Geometry: final body of the model. Coordinates: model frame, mm. A direction names the side the tool comes from. Round coordinates to 2 decimals unless told otherwise and drop trailing zeros. Answer in a Markdown table with one row per item.
Autodesk Inventor part; units mm, degrees
ref_plane "C1_XY" through (0, 0, 0) normal (0, 0, 1) x (1, 0, 0)
ref_plane "C1_YZ" through (0, 0, 0) normal (1, 0, 0) x (0, 1, 0)
ref_plane "C1_ZX" through (0, 0, 0) normal (0, 1, 0) x (0, 0, 1)
sketch "Sketch_63" plane through (0, 0, 0) normal (0, 0, 1) x (1, 0, 0)
  line L0 (-10, -7) -> (-8, -7)
  line L1 (-8, -7) -> (-8, -4)
  line L2 (-8, -4) -> (-7.0607, -4)
  line L3 (-7.0607, -4) -> (-4, -7.0607)
  line L4 (-4, -7.0607) -> (-4, -9.4804)
  line L5 (-4, -9.4804) -> (-3.7, -10)
  line L6 (-3.7, -10) -> (-4, -10.5196)
  line L7 (-4, -10.5196) -> (-4, -12.9393)
  line L8 (-4, -12.9393) -> (-7.0607, -16)
  line L9 (-7.0607, -16) -> (-8, -16)
  line L10 (-8, -16) -> (-8, -13)
  line L11 (-8, -13) -> (-10, -13)
  line L12 (-10, -13) -> (-10, -19)
  arc A0 (-10, -19) -> (-9, -20) centre (-9, -19) ccw
  line L13 (-9, -20) -> (-3, -20)
  line L14 (-3, -20) -> (-3, -18)
  line L15 (-3, -18) -> (-6, -18)
  line L16 (-6, -18) -> (-6, -17.0607)
  line L17 (-6, -17.0607) -> (-2.9393, -14)
  line L18 (-2.9393, -14) -> (-0.5196, -14)
  line L19 (-0.5196, -14) -> (0, -13.7)
  line L20 (0, -13.7) -> (0.5196, -14)
  line L21 (0.5196, -14) -> (2.9393, -14)
  line L22 (2.9393, -14) -> (6, -17.0607)
  line L23 (6, -17.0607) -> (6, -18)
  line L24 (6, -18) -> (3, -18)
  line L25 (3, -18) -> (3, -20)
  line L26 (3, -20) -> (9, -20)
  arc A1 (9, -20) -> (10, -19) centre (9, -19) ccw
  line L27 (10, -19) -> (10, 19)
  arc A2 (10, 19) -> (9, 20) centre (9, 19) ccw
  line L28 (9, 20) -> (3, 20)
  line L29 (3, 20) -> (3, 18)
  line L30 (3, 18) -> (6, 18)
  line L31 (6, 18) -> (6, 17.0607)
  line L32 (6, 17.0607) -> (2.9393, 14)
  line L33 (2.9393, 14) -> (0.5196, 14)
  line L34 (0.5196, 14) -> (0, 13.7)
  line L35 (0, 13.7) -> (-0.5196, 14)
  line L36 (-0.5196, 14) -> (-2.9393, 14)
  line L37 (-2.9393, 14) -> (-6, 17.0607)
  line L38 (-6, 17.0607) -> (-6, 18)
  line L39 (-6, 18) -> (-3, 18)
  line L40 (-3, 18) -> (-3, 20)
  line L41 (-3, 20) -> (-9, 20)
  arc A3 (-9, 20) -> (-10, 19) centre (-9, 19) ccw
  line L42 (-10, 19) -> (-10, 13)
  line L43 (-10, 13) -> (-8, 13)
  line L44 (-8, 13) -> (-8, 16)
  line L45 (-8, 16) -> (-7.0607, 16)
  line L46 (-7.0607, 16) -> (-4, 12.9393)
  line L47 (-4, 12.9393) -> (-4, 10.5196)
  line L48 (-4, 10.5196) -> (-3.7, 10)
  line L49 (-3.7, 10) -> (-4, 9.4804)
  line L50 (-4, 9.4804) -> (-4, 7.0607)
  line L51 (-4, 7.0607) -> (-7.0607, 4)
  line L52 (-7.0607, 4) -> (-8, 4)
  line L53 (-8, 4) -> (-8, 7)
  line L54 (-8, 7) -> (-10, 7)
  line L55 (-10, 7) -> (-10, -7)
  line L56 (4, 12.9393) -> (4, 8.5)
  arc A4 (4, 8.5) -> (5, 7.5) centre (5, 8.5) ccw
  line L57 (5, 7.5) -> (7, 7.5)
  arc A5 (7, 7.5) -> (8, 8.5) centre (7, 8.5) ccw
  line L58 (8, 8.5) -> (8, 16)
  line L59 (8, 16) -> (7.0607, 16)
  line L60 (7.0607, 16) -> (4, 12.9393)
  line L61 (4, -12.9393) -> (7.0607, -16)
  line L62 (7.0607, -16) -> (8, -16)
  line L63 (8, -16) -> (8, -8.5)
  arc A6 (8, -8.5) -> (7, -7.5) centre (7, -8.5) ccw
  line L64 (7, -7.5) -> (5, -7.5)
  arc A7 (5, -7.5) -> (4, -8.5) centre (5, -8.5) ccw
  line L65 (4, -8.5) -> (4, -12.9393)
  line L66 (-8, 1.7) -> (-8, -1.7)
  arc A8 (-8, -1.7) -> (-7.7, -2) centre (-7.7, -1.7) ccw
  line L67 (-7.7, -2) -> (-7.0636, -2)
  arc A9 (-6.8515, -2.0879) -> (-7.0636, -2) centre (-7.0636, -2.3) ccw
  line L68 (-6.8515, -2.0879) -> (-2.9393, -6)
  line L69 (-2.9393, -6) -> (7, -6)
  arc A10 (7, -6) -> (8, -5) centre (7, -5) ccw
  line L70 (8, -5) -> (8, 5)
  arc A11 (8, 5) -> (7, 6) centre (7, 5) ccw
  line L71 (7, 6) -> (-2.9393, 6)
  line L72 (-2.9393, 6) -> (-6.8515, 2.0879)
  arc A12 (-7.0636, 2) -> (-6.8515, 2.0879) centre (-7.0636, 2.3) ccw
  line L73 (-7.0636, 2) -> (-7.7, 2)
  arc A13 (-7.7, 2) -> (-8, 1.7) centre (-7.7, 1.7) ccw
extrude "Extrusion1" add sketch "Sketch_63" against normal blind 500
sketch "Sketch2" plane through (0, 0, -500) normal (0, 0, -1) x (-1, 0, 0)
  point P0 (0, 10)
hole "Hole1" at (0, 10, -500) direction (0, 0, 1) diameter 4.2 end through all
pattern_linear "Rectangular Pattern1" count 2 spacing 20 along (0, -1, 0) of "Hole1"
ref_plane "C1_XY" through (0, 0, 0) normal (0, 0, 1) x (1, 0, 0)
ref_plane "C1_YZ" through (0, 0, 0) normal (1, 0, 0) x (0, 1, 0)
ref_plane "C1_ZX" through (0, 0, 0) normal (0, 1, 0) x (0, 0, 1)
thread "Thread1"
thread "Thread2"
thread "Thread3"
thread "Thread4"
properties part number "HFSF5-2040-500" material "Aluminum 6061"
Item 1: Cut plane A-A (z = -250.5). Count the separate pieces of the cut face and the enclosed holes in it, then the cut area to 3 significant figures.
Answer:
| item | result |
|---|---|
| separate pieces | 1 |
| enclosed holes | 5 |
| area | 343 mm² |
Item 2: Reachability of faces 1 (the face through (-5, 5, -500)), 2 (the face through (8, 0, -246)) from +Z, -Z, +X, -X, +Y, -Y: full face, straight path, thin tool, end or side. Return the list, or none.
Answer:
| item | result |
|---|---|
| face 1 | -Z, +X, -X, +Y, -Y |
| face 2 | +Z, -Z |
Item 3: Pin query (flat end, axial travel): pin 1 Ø1.2 at (x, z) = (2, -195.5) entering from +Y; pin 2 Ø0.7 at (x, z) = (-2, -240) entering from -Y; pin 3 Ø0.7 at (y, z) = (9, -156.5) entering from -X; pin 4 Ø3.5 at (x, y) = (0, -10) entering from +Z. Return the tip coordinate at first contact, or that it passes through.
Answer:
| item | result |
|---|---|
| pin 1 | stops at y = 14 |
| pin 2 | stops at y = -14 |
| pin 3 | stops at x = -4 |
| pin 4 | passes through |
Item 4: Draft query along Y for faces 3 (the face through (10, 0, -246)), 4 (the face through (2, 6, -246)). Return one class per face: pulls with the +Y half, pulls with the -Y half, needs draft (parallel to the pull), parting line crosses it, or undercut.
Answer:
| item | result |
|---|---|
| face 3 | needs draft |
| face 4 | undercut |
Item 5: Line query: probe 1 along X at (y, z) = (-10, -369.5); probe 2 along X at (y, z) = (9.5, -51); probe 3 along Y at (x, z) = (0.5, -147.5). Output: solid intervals per line, ascending. Write a range as [from, to].
Answer:
| item | result |
|---|---|
| probe 1 | x = [-3.7, -2.1], [2.1, 4], [8, 10] |
| probe 2 | x = [-3.99, -2.04], [2.04, 4], [8, 10] |
| probe 3 | y = [-13.99, -12.04], [-7.96, -6], [6, 7.96], [12.04, 13.99] |
